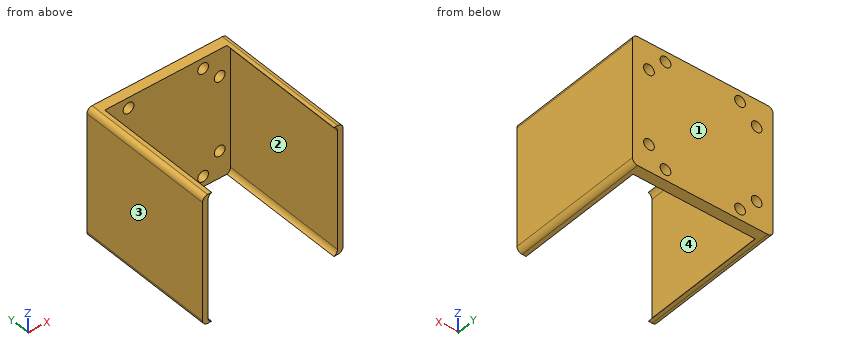
Autodesk Inventor part; units mm, degrees
ref_plane "Work Plane1" through (124.725, 49.8, -24.875) normal (0, 1, 0) x (0, 0, 1)
ref_plane "Work Plane2" through (149.6, 49.8, -22.9) normal (-1, 0, 0) x (0, 0, 1)
ref_plane "YZ Plane" through (0, 0, 0) normal (1, 0, 0) x (0, 1, 0)
sketch "Sketch1" plane through (0, 0, 0) normal (0, 1, 0) x (-1, 0, 0)
  line L0 (-155.225, -15) -> (-155.225, 15)
  line L1 (-155.225, 15) -> (-147.725, 15)
  line L2 (-147.725, 15) -> (-147.725, -15)
  line L3 (-147.725, -15) -> (-155.225, -15)
  circle A0 centre (-171.5, -21.9) radius 1.875
  circle A1 centre (-127.7, 21.9) radius 1.875
  circle A2 centre (-127.7, -21.9) radius 1.875
  circle A3 centre (-171.5, 21.9) radius 1.875
  circle A4 centre (-135.2, 20.8) radius 2.0734
  circle A5 centre (-164, -20.8) radius 2.0734
  circle A6 centre (-135.2, -20.8) radius 2.0734
  circle A7 centre (-128.8, -14.4) radius 2.0734
  circle A8 centre (-128.8, 14.4) radius 2.0734
  circle A9 centre (-164, 20.8) radius 2.0734
  circle A10 centre (-170.4, -14.4) radius 2.0734
  circle A11 centre (-170.4, 14.4) radius 2.0734
  line L4 (-172.5, 24.875) -> (-126.7, 24.875)
  arc A12 (-172.5, 24.875) -> (-174.475, 22.9) centre (-172.5, 22.9) ccw
  line L5 (-174.475, -22.9) -> (-174.475, 22.9)
  arc A13 (-174.475, -22.9) -> (-172.5, -24.875) centre (-172.5, -22.9) ccw
  line L6 (-126.7, -24.875) -> (-172.5, -24.875)
  arc A14 (-126.7, -24.875) -> (-124.725, -22.9) centre (-126.7, -22.9) ccw
  line L7 (-124.725, 22.9) -> (-124.725, -22.9)
  arc A15 (-124.725, 22.9) -> (-126.7, 24.875) centre (-126.7, 22.9) ccw
  point P0 (0, 0)
ref_plane "Work Plane1" through (124.725, 49.8, -24.875) normal (0, 1, 0) x (0, 0, 1)
extrude "Extrusion1" add sketch "Sketch1" along normal blind 4 from surface at 49.8 contours L0 L1 L2 L3 | A0 | A1 | A2 | A3 | L4 A15 L7 A14 L6 A13 L5 A12
sketch "Sketch2" plane through (126.7, 53.8, -24.875) normal (0, 1, 0) x (1, 0, 0)
  circle A0 centre (8.5, -45.675) radius 2.0734
  circle A1 centre (37.3, -4.075) radius 2.0734
  circle A2 centre (8.5, -4.075) radius 2.0734
  circle A3 centre (2.1, -10.475) radius 2.0734
  circle A4 centre (2.1, -39.275) radius 2.0734
  circle A5 centre (37.3, -45.675) radius 2.0734
  circle A6 centre (43.7, -10.475) radius 2.0734
  circle A7 centre (43.7, -39.275) radius 2.0734
  arc A8 (47.775, -1.975) -> (45.8, 0) centre (45.8, -1.975) ccw
  line L0 (0, 0) -> (45.8, 0)
  arc A9 (0, 0) -> (-1.975, -1.975) centre (0, -1.975) ccw
  line L1 (-1.975, -47.775) -> (-1.975, -1.975)
  arc A10 (-1.975, -47.775) -> (0, -49.75) centre (0, -47.775) ccw
  line L2 (45.8, -49.75) -> (0, -49.75)
  arc A11 (45.8, -49.75) -> (47.775, -47.775) centre (45.8, -47.775) ccw
  line L3 (47.775, -1.975) -> (47.775, -47.775)
  line L4 (16.025, -44.875) -> (33.525, -44.875)
  line L5 (33.525, -44.875) -> (33.525, -4.875)
  line L6 (33.525, -4.875) -> (16.025, -4.875)
  line L7 (16.025, -4.875) -> (16.025, -44.875)
  line L8 (45.8, 0) -> (50.05, 0)
  line L9 (50.05, 0) -> (50.05, -49.75)
  line L10 (50.05, -49.75) -> (45.8, -49.75)
  line L11 (45.8, -49.75) -> (45.8, 0)
  line L12 (50.05, -49.75) -> (47.925, -49.75)
  line L13 (47.925, -49.75) -> (47.925, 0)
  line L14 (47.925, 0) -> (50.05, 0)
  line L15 (50.05, 0) -> (50.05, -49.75)
  arc A12 (45.8, -49.875) -> (47.9, -47.775) centre (45.8, -47.775) ccw
  line L16 (45.8, -49.875) -> (0, -49.875)
  arc A13 (-2.1, -47.775) -> (0, -49.875) centre (0, -47.775) ccw
  line L17 (-2.1, -47.775) -> (-2.1, -1.975)
  arc A14 (0, 0.125) -> (-2.1, -1.975) centre (0, -1.975) ccw
  line L18 (0, 0.125) -> (45.8, 0.125)
  arc A15 (47.9, -1.975) -> (45.8, 0.125) centre (45.8, -1.975) ccw
  line L19 (47.9, -1.975) -> (47.9, -47.775)
  point P0 (-126.7, -24.875)
  point P1 (47.925, -49.75)
  point P2 (46.5137, -49.75)
  point P3 (46.5137, 0)
  dimension "d3" = 4.25
  dimension "d4" = 2.125
  dimension "d15" = 0.125
extrude "Extrusion2" [suppressed]
extrude "Extrusion3" add sketch "Sketch2" against normal up to surface (4 mm away) contours A8 L8 A15 L19 A12 L10 A11 L3 | L8 L13 L10 A12 L19 A15 | L8 L9 L10 L13
extrude "Extrusion4" add sketch "Sketch2" against normal blind 49.8 from surface at -4 contours L8 L13 L10 A12 L19 A15 | L8 L9 L10 L13
fillet "Fillet1" radius 2 2 edges at (176.75, 26.9, 24.875) (176.75, 26.9, -24.875)
sketch "Sketch3" plane through (176.75, 53.8, 22.875) normal (1, 0, 0) x (0, 0, -1)
  line L0 (7.875, -21.425) -> (7.875, -28.925)
  line L1 (7.875, -28.925) -> (37.875, -28.925)
  line L2 (37.875, -28.925) -> (37.875, -21.425)
  line L3 (37.875, -21.425) -> (7.875, -21.425)
  line L4 (5.825, -9.7) -> (39.925, -9.7)
  line L5 (39.925, -44.1) -> (39.925, -9.7)
  line L6 (5.825, -44.1) -> (39.925, -44.1)
  line L7 (5.825, -9.7) -> (5.825, -44.1)
  line L8 (2.875, -16.425) -> (2.875, -33.925)
  line L9 (2.875, -33.925) -> (42.875, -33.925)
  line L10 (42.875, -33.925) -> (42.875, -16.425)
  line L11 (42.875, -16.425) -> (2.875, -16.425)
  point P0 (22.875, -53.8)
  dimension "d12" = 5
extrude "Extrusion5" [suppressed]
ref_plane "Work Plane2" through (149.6, 49.8, -22.9) normal (-1, 0, 0) x (0, 0, 1)
mirror "Mirror1" about plane through (149.6, 49.8, -22.9) normal (-1, 0, 0) of "Extrusion3", "Extrusion4", "Fillet1"
properties part number "Outer Cover Full"
Source: CAD feature listing. Evaluate the final solid. Frame: model axes, mm. Face numbers are marked on the shaded views. A direction names the side the tool comes from. Coordinates: 2 decimals unless noted, no trailing zeros. Write each loop counter-clockwise with the first axis right and the second up, starting at its lowest first coordinate (ties: lowest second). Pieces come first, ordered by that corner, then holes. Notation, with made-up numbers: (6.25, -32) - (35.25, -32) arc R19 cw to (35.25, -28) - close; hole circle Ø4 at (-26.5, 64). An arc over 180 degrees is marked (long way). Answer as a JSON object with one key per item and string values.
Q1. Section query B-B, the plane y = 28. Output: boundary loops of the cut face in (x, z) (3 decimals), plus the area to 3 significant figures.
Ans:
{"outline": "(122.45, -22.875) arc R2 ccw to (124.45, -24.875) - (125.986, -24.875) arc R2.1 cw to (124.6, -22.9) - (124.6, 22.9) arc R2.1 cw to (125.986, 24.875) - (124.45, 24.875) arc R2 ccw to (122.45, 22.875) - close; (173.214, -24.875) - (174.75, -24.875) arc R2 ccw to (176.75, -22.875) - (176.75, 22.875) arc R2 ccw to (174.75, 24.875) - (173.214, 24.875) arc R2.1 cw to (174.6, 22.9) - (174.6, -22.9) arc R2.1 cw to start", "area": "213 mm2"}
Q2. Draft query along Z for the marked faces 1 and 2. Return one class per face: released by +Z, released by -Z, zero draft, split by the parting line, or undercut.
Ans:
{"face 1": "zero draft", "face 2": "undercut"}
Q3. Section query A-A, the plane x = 135.2. Output: boundary loops of the cut face in (y, z) (3 decimals), plus the area to 3 significant figures.
Ans:
{"outline": "(49.8, -24.875) - (53.8, -24.875) - (53.8, -22.873) - (49.8, -22.873) - close; (49.8, -18.727) - (53.8, -18.727) - (53.8, 18.727) - (49.8, 18.727) - close; (49.8, 22.873) - (53.8, 22.873) - (53.8, 24.875) - (49.8, 24.875) - close", "area": "166 mm2"}
Q4. Section query D-D, the plane x = 156.5. Output: boundary loops of the cut face in (y, z) (3 decimals), plus the area to 3 significant figures.
Ans:
{"outline": "(49.8, -24.875) - (53.8, -24.875) - (53.8, 24.875) - (49.8, 24.875) - close", "area": "199 mm2"}
Q5. Material intervals for line 1 (Z direction, x = 135, y = 52) (3 decimals); line 2 (X direction, y = 41, z = 16); line 3 (Z direction, x = 128.8, y = 51.35) (3 decimals), sorted ascending. Write a range as [from, to].
Ans:
{"line 1": "z = [-24.875, -22.864], [-18.736, 18.736], [22.864, 24.875]", "line 2": "x = [122.45, 124.6], [174.6, 176.75]", "line 3": "z = [-24.875, -16.473], [-12.327, 12.327], [16.473, 24.875]"}
Q6. Set-up query: the marked faces 3 and 4. Return all of +Z, -Z, +X, -X, +Y, -Y with unobstructed straight access to the full face (end or side cutting, diameter ignored); none if empty.
Ans:
{"face 3": "+Z, -Z, -X, +Y, -Y", "face 4": "-Y"}
Q7. Section query C-C, the plane z = 14.4. Output: boundary loops of the cut face in (x, y).
Ans:
{"outline": "(122.45, 0) - (124.6, 0) - (124.6, 49.8) - (126.73, 49.8) - (126.73, 53.8) - (122.45, 53.8) - close; (130.87, 49.8) - (168.33, 49.8) - (168.33, 53.8) - (130.87, 53.8) - close; (172.47, 49.8) - (174.6, 49.8) - (174.6, 0) - (176.75, 0) - (176.75, 53.8) - (172.47, 53.8) - close"}
Q8. First-contact query: pin 1 Ø6 at (x, z) = (152.5, 12.5) entering from -Y. Flat tip, straight axial feed; report the tip coordinate or a pass-through.
Ans:
{"pin 1": "stops at y = 49.8"}
